```python
from build123d import *

# Parameters (mm, degrees)
F0_R        = 2.5
F1_DEPTH    = 10
F2_R        = 1.5
F3_DEPTH    = 25
F4_R        = 1.99999
F5_T1_DEPTH = 19.6824712753
F6_R        = 5
F7_R        = 2
F8_R        = 1.99999
F9_SIZE     = 0.49999
F10_SIZE    = 0.5


# Not quite as in the source:
# - a fillet or chamfer that OpenCascade refuses, or shapes differently, is made with other operations: its cross-section is extruded or revolved along the edge and cut away or added
# - a fillet or chamfer is up to 0.001 mm smaller than in the source, because OpenCascade refuses the exact size


with BuildPart() as f1:
    # F0 (on Front) → F1 (new body)
    with BuildSketch(Plane.XZ):
        Polygon((-2.75, 9.5), (-6.25, 9.5), (-6.25, -5.5), (16.25, -5.5), (16.25, -1.5), (6.25, -1.5), (6.25, 5.5), (-3.25, 5.5), (-3.25, 7), (-2.75, 7.5), align=None)
        Circle(F0_R, mode=Mode.SUBTRACT)
    extrude(amount=F1_DEPTH)

    # F2 (on face) → F3 (cut)
    with BuildSketch(Plane.XY.offset(-1.5)):
        with Locations((11.25, -8)):
            Circle(F2_R)
        with Locations((11.25, -2)):
            Circle(F2_R)
    extrude(amount=-F3_DEPTH, mode=Mode.SUBTRACT)

    # F4 (radius 2 in the source; OpenCascade refuses exactly that, so slightly less here)
    f4_edges = [f1.edges().sort_by_distance(p)[0] for p in [
        (-2.75, -5, 9.5),
    ]]
    fillet(f4_edges, radius=F4_R)

    # F5: fillet of radius 2 on 1 edges, made by hand

    # F5_s2 → F5_t1 (cut)
    with BuildSketch(Plane.XZ.offset(-4.8412356377)):
        with BuildLine():
            ThreePointArc((-4.74999, 9.5), (-5.8311356678, 8.7882546988), (-6.25, 7.5635057449))
            Line((-6.25, 7.5635057449), (-6.25, 9.5))
            Line((-6.25, 9.5), (-4.74999, 9.5))
        make_face()
    extrude(amount=F5_T1_DEPTH, mode=Mode.SUBTRACT)

    # F6
    f6_edges = [f1.edges().sort_by_distance(p)[0] for p in [
        (-6.25, -5, -5.5),
    ]]
    fillet(f6_edges, radius=F6_R)

    # F7
    f7_edges = [f1.edges().sort_by_distance(p)[0] for p in [
        (6.25, -5, 5.5),
    ]]
    fillet(f7_edges, radius=F7_R)

    # F8 (radius 2 in the source; OpenCascade refuses exactly that, so slightly less here)
    f8_edges = [f1.edges().sort_by_distance(p)[0] for p in [
        (16.25, -5, -1.5),
        (16.25, -5, -5.5),
    ]]
    fillet(f8_edges, radius=F8_R)

    # F9 (size 0.5 in the source; OpenCascade refuses exactly that, so slightly less here)
    f9_edges = [f1.edges().sort_by_distance(p)[0] for p in [
        (9.75, -8, -5.5),
        (9.75, -2, -5.5),
    ]]
    chamfer(f9_edges, length=F9_SIZE)

    # F10
    f10_edges = [f1.edges().sort_by_distance(p)[0] for p in [
        (-2.5, -10, 0),
        (-2.5, 0, 0),
    ]]
    chamfer(f10_edges, length=F10_SIZE)


solid = f1.part
```
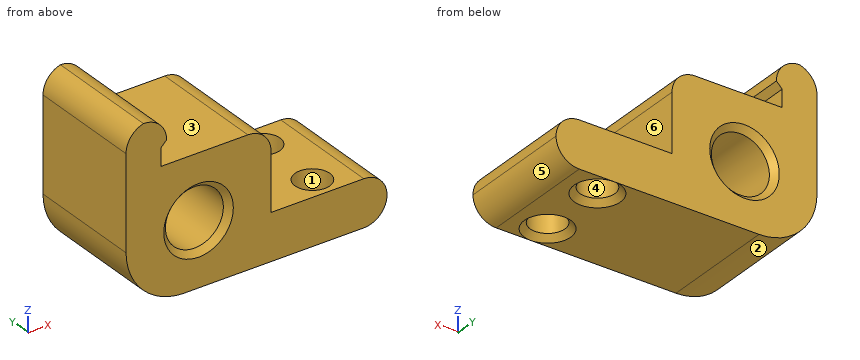
Input: part model. Units: mm. Frame: model coordinates. Face numbers are marked on the shaded views. A direction names the side the tool comes from. Coordinates: 2 decimals unless noted, no trailing zeros. Order: outer loops, then holes, each group sorted by start corner. A loop starts at its lowest first (then second) coordinate and runs counter-clockwise, first axis right, second up. Notation, with made-up numbers: (59.5, 49) - (113.5, 49) arc R14 ccw to (113.5, 63) - close; hole circle Ø7 at (6, -13). An arc over 180 degrees is marked (long way). Put each result on its own line as item: value.
1. Reachability of the marked faces 5 and 6 from +Z, -Z, +X, -X, +Y, -Y: full face, straight path, thin tool, end or side. Return the list, or none.
Report:
face 5: -Z, +X, +Y, -Y
face 6: +Z, +X, +Y, -Y
2. Contact query for flat-ended pins moving along their axis: pin 1 Ø5.5 at (y, z) = (-5.5, 0) entering from +X; pin 2 Ø5 at (x, y) = (-2, -5.5) entering from +Z; pin 3 Ø3 at (y, z) = (-3.5, -1) entering from +X; pin 4 Ø5 at (x, y) = (11.25, -8) entering from -Z. Output: stop coordinate, or through.
Report:
pin 1: stops at x = 16.1
pin 2: stops at z = 9.48
pin 3: stops at x = 15.98
pin 4: stops at z = -5.5
3. Draft query along X for the marked faces 1, 2, 3 and 4. Return one class per face: pulls with the +X half, pulls with the -X half, needs draft (parallel to the pull), parting line crosses it, or undercut.
Report:
face 1: undercut
face 2: pulls with the -X half
face 3: needs draft
face 4: undercut
4. Cut plane A-A on y = -2. State how many separate pieces and enclosed holes the cut face has, then the cut area to 3 significant figures.
Report:
separate pieces: 2
enclosed holes: 1
area: 149 mm2
5. Cut plane C-C on z = 0. Return the cut outline in (x, y).
Report:
outline: (-6.25, -10) - (-3, -10) - (-2.5, -9.5) - (-2.5, -0.5) - (-3, 0) - (-6.25, 0) - close; (2.5, -9.5) - (3, -10) - (6.25, -10) - (6.25, 0) - (3, 0) - (2.5, -0.5) - close
6. Line query: line 1 along Y through (x, z) = (11.25, -4); line 2 along Z through (x, y) = (10, -5); line 3 along Z through (x, y) = (0.5, -9.25). Output: solid intervals per line, ascending.
Report:
line 1: y = -10 to -9.5, -6.5 to -3.5, -0.5 to 0
line 2: z = -5.5 to -1.5
line 3: z = -5.5 to -2.45, 2.45 to 5.5
